Check sheet for the drawn part. Datum: minimum x, y, z corner. Units: mm. A direction names the side the tool comes from. Coordinates: 2 decimals unless noted, no trailing zeros. Order: outer loops, then holes, each group sorted by start corner. A loop starts at its lowest first (then second) coordinate and runs counter-clockwise, first axis right, second up.
Q1. Cross-section at C-C, the plane z = 5.25. Record the boundary of the cut face in (x, y) (3 decimals).
Q2. Cross-section at B-B, the plane y = 6.5. Record the boundary of the cut face in (x, z), and give its area (3 significant figures).
Q3. Depth check by flat-ended pin: P1, Ø3, axis at y = 5.5, z = 4, coming from the +X side; P2, Ø2, axis at x = 18.75, y = 5.275, coming from the +Z side; P3, Ø0.7, axis at x = 0.5, z = 2, coming from the -Y side; P4, Ø2.5, axis at y = 5, z = 3.5, coming from the -X side. Enter the tip coordinate at first touch or a pass-through.
Q4. Thickness scan on line 1 (Y direction, x = 18.75, z = 5.25) (3 decimals); line 2 (Y direction, x = 22.75, z = 3.75); line 3 (X direction, y = 6, z = 1.5). Record the ranges inside material, lowest first.
Q5. Draft check along X on the marked faces 1, 2 and 3. Enter one of: pulls with the +X half, pulls with the -X half, needs draft (parallel to the pull), parting line crosses it, or undercut.
Q6. Cross-section at D-D, the plane x = 18.75. Record the boundary of the cut face in (y, z) (3 decimals), and give its area (3 significant figures).
Q7. Cross-section at A-A, the plane x = 8.75. Record the boundary of the cut face in (y, z), and give its area (3 significant figures).
Q8. Set-up check for the marked faces 4, 5, 6 and 7: record each of +Z, -Z, +X, -X, +Y, -Y from which the full face is reachable in a straight line by a thin tool's end or side.
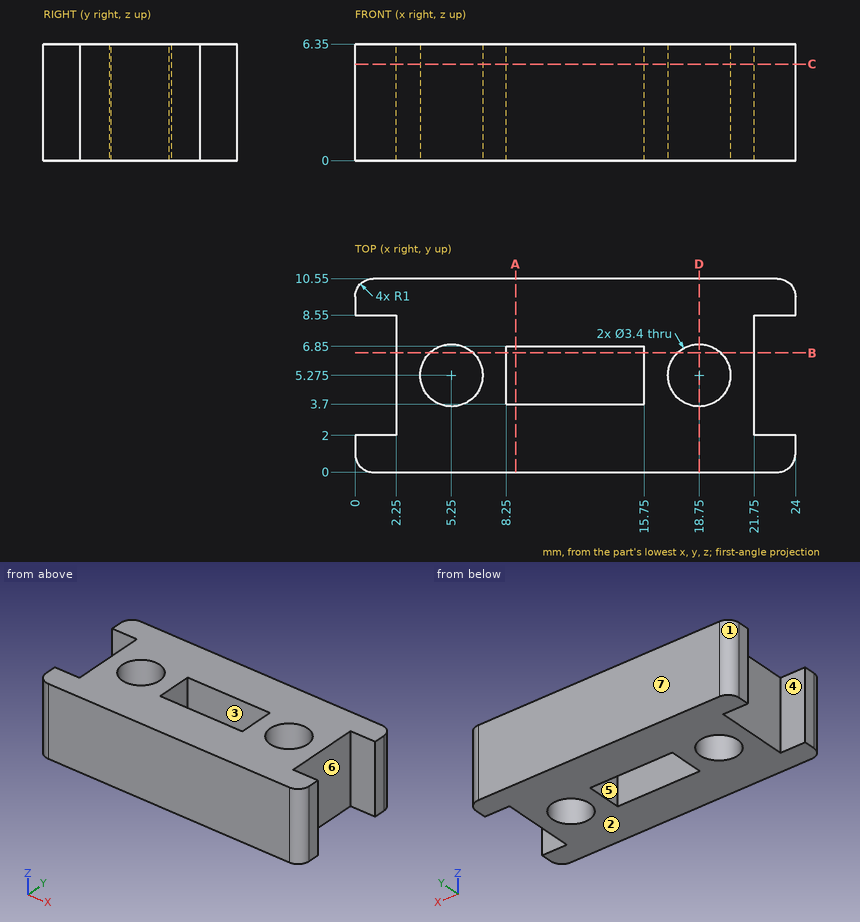
Check values:
1. outline: (0, 1) arc R1 ccw to (1, 0) - (23, 0) arc R1 ccw to (24, 1) - (24, 2) - (21.75, 2) - (21.75, 8.55) - (24, 8.55) - (24, 9.55) arc R1 ccw to (23, 10.55) - (1, 10.55) arc R1 ccw to (0, 9.55) - (0, 8.55) - (2.25, 8.55) - (2.25, 2) - (0, 2) - close; hole circle Ø3.4 at (5.25, 5.275); hole (8.25, 3.7) - (15.75, 3.7) - (15.75, 6.85) - (8.25, 6.85) - close; hole circle Ø3.4 at (18.75, 5.275)
2. outline: (2.25, 0) - (4.07, 0) - (4.07, 6.35) - (2.25, 6.35) - close; (6.43, 0) - (8.25, 0) - (8.25, 6.35) - (6.43, 6.35) - close; (15.75, 0) - (17.57, 0) - (17.57, 6.35) - (15.75, 6.35) - close; (19.93, 0) - (21.75, 0) - (21.75, 6.35) - (19.93, 6.35) - close
2. area: 46.3 mm2
3. P1: stops at x = 21.75
3. P2: passes through
3. P3: stops at y = 0.01
3. P4: stops at x = 2.25
4. line 1: y = 0 to 3.575, 6.975 to 10.55
4. line 2: y = 0 to 2, 8.55 to 10.55
4. line 3: x = 2.25 to 3.71, 6.79 to 8.25, 15.75 to 17.21, 20.29 to 21.75
5. face 1: pulls with the -X half
5. face 2: needs draft
5. face 3: undercut
6. outline: (0, 0) - (3.575, 0) - (3.575, 6.35) - (0, 6.35) - close; (6.975, 0) - (10.55, 0) - (10.55, 6.35) - (6.975, 6.35) - close
6. area: 45.4 mm2
7. outline: (0, 0) - (3.7, 0) - (3.7, 6.35) - (0, 6.35) - close; (6.85, 0) - (10.55, 0) - (10.55, 6.35) - (6.85, 6.35) - close
7. area: 47.0 mm2
8. face 4: +Z, -Z, -X
8. face 5: +Z, -Z
8. face 6: +Z, -Z, +X
8. face 7: +Z, -Z, +X, -X, +Y
